Can you work these out from the model? Positions are in its coordinate system, mm. Face numbers are marked on the shaded views. Round coordinates to 2 decimals unless told otherwise and drop trailing zeros. Order: outer loops, then holes, each group sorted by start corner. A loop starts at its lowest first (then second) coordinate and runs counter-clockwise, first axis right, second up.
Q1. If we section it at A-A (x = 0): Please give me the cut outline in (y, z).
Q2. If I drill on line 1 (Y direction, x = 0, z = -13); line 2 (X direction, y = 76, z = -30); line 3 (Y direction, x = 44.5, z = -2.5), over which ranges is the centre line in solid material (lowest first)?
Q3. If we section it at B-B (y = 51): Please give me the cut outline in (x, z).
Q4. If we section it at C-C (z = 36): Please give me the cut outline in (x, y).
Q5. We'd pull the mould along X, two halves only. Please class the marked faces 1, 2, 3 and 4: pulls with the +X half, pulls with the -X half, needs draft (parallel to the pull), parting line crosses it, or undercut.
from build123d import *

# Parameters (mm, degrees)
F0_W     = 152.4
F0_H     = 152.4
F1_DEPTH = 152.4
F2_R     = 63.5
F3_DEPTH = 152.401


with BuildPart() as f1:
    # F0 (on Front) → F1 (new body)
    with BuildSketch(Plane.XZ):
        Rectangle(F0_W, F0_H)
    extrude(amount=-F1_DEPTH)

    # F2 (on face) → F3 (cut, through all)
    with BuildSketch(Plane.XY.offset(76.2)):
        with Locations((0, 76.2)):
            Circle(F2_R)
    extrude(amount=-F3_DEPTH, mode=Mode.SUBTRACT)


solid = f1.part
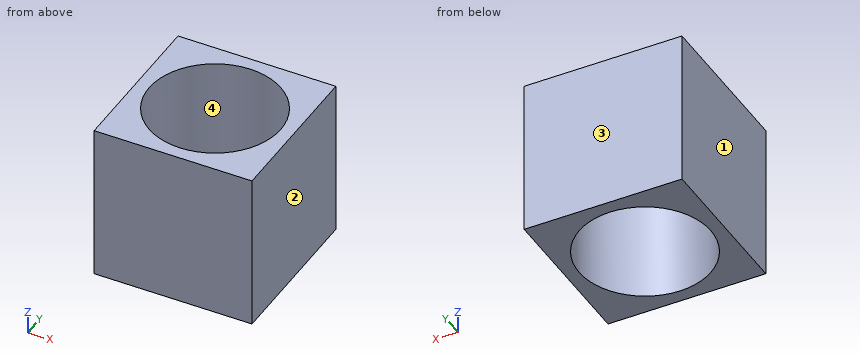
Solution:
1. outline: (0, -76.2) - (12.7, -76.2) - (12.7, 76.2) - (0, 76.2) - close; (139.7, -76.2) - (152.4, -76.2) - (152.4, 76.2) - (139.7, 76.2) - close
2. line 1: y = 0 to 12.7, 139.7 to 152.4
2. line 2: x = -76.2 to -63.5, 63.5 to 76.2
2. line 3: y = 0 to 30.9, 121.5 to 152.4
3. outline: (-76.2, -76.2) - (-58.29, -76.2) - (-58.29, 76.2) - (-76.2, 76.2) - close; (58.29, -76.2) - (76.2, -76.2) - (76.2, 76.2) - (58.29, 76.2) - close
4. outline: (-76.2, 0) - (76.2, 0) - (76.2, 152.4) - (-76.2, 152.4) - close; hole circle Ø127 at (0, 76.2)
5. face 1: pulls with the -X half
5. face 2: pulls with the +X half
5. face 3: needs draft
5. face 4: undercut
